Source: CAD feature listing. Evaluate the final solid. Frame: model axes, mm. A direction names the side the tool comes from. Round coordinates to 2 decimals unless told otherwise and drop trailing zeros. Loops run counter-clockwise (first coordinate to the right, second up) from the corner with the lowest first, then second, coordinate; pieces in that order, holes last. Notation, with made-up numbers: (70.5, 82) -> (127.5, 82) arc R20 cw to (127.5, 99) -> close; hole circle Ø1 at (48, 49.25). An arc over 180 degrees is marked (long way). Write item = value, one per line.
from build123d import *

# Parameters (mm, degrees)
F0_W     = 100
F0_H     = 300
F1_DEPTH = 6.35
F2_W     = 2
F2_H     = 40
F3_DEPTH = 25.4


# Not quite as in the source:
# - a length typed as a fraction of an inch, garbled in the dataset ("3 / 203.2 mm" for 3/8 in), is restored


with BuildPart() as f1:
    # F0 (on Top) → F1 (new body)
    with BuildSketch(Plane.XY):
        Rectangle(F0_W, F0_H)
    extrude(amount=F1_DEPTH)

    # F2 (on face) → F3 (cut)
    with BuildSketch(Plane.XY.offset(6.35)):
        Polygon((22.5, 22.48), (22.5, 110.5), (-22.5, 110.5), (-22.5, 22.48), (-22.5, -17.52), (-22.5, -110.5), (22.5, -110.5), (22.5, -17.52), align=None)
        with Locations((23.5, 2.48)):
            Rectangle(F2_W, F2_H)
        with Locations((-23.5, 2.48)):
            Rectangle(F2_W, F2_H)
    extrude(amount=-F3_DEPTH, mode=Mode.SUBTRACT)


solid = f1.part
1. Contact query for a flat-ended pin moving along its axis: pin 1 Ø1.5 at (x, y) = (22.5, 17) entering from -Z. Output: stop coordinate, or through.
Evaluation:
pin_1 = through
2. Section query C-C (z = 4). Return the cut outline in (x, y).
Evaluation:
outline = (-50, -150) -> (50, -150) -> (50, 150) -> (-50, 150) -> close; hole (-24.5, -17.52) -> (-22.5, -17.52) -> (-22.5, -110.5) -> (22.5, -110.5) -> (22.5, -17.52) -> (24.5, -17.52) -> (24.5, 22.48) -> (22.5, 22.48) -> (22.5, 110.5) -> (-22.5, 110.5) -> (-22.5, 22.48) -> (-24.5, 22.48) -> close
3. Section query B-B (y = 37). Return the cut outline in (x, z), then the cut area to 3 significant figures.
Evaluation:
outline = (-50, 0) -> (-22.5, 0) -> (-22.5, 6.35) -> (-50, 6.35) -> close; (22.5, 0) -> (50, 0) -> (50, 6.35) -> (22.5, 6.35) -> close
area = 349 mm²
4. Mould query, pull axis X, two halves, no side actions, for faces 1 (the face through (50, -2, 3)), 2 (the face through (-34, 2, 0)), 3 (the face through (-22.5, 67, 3)). Classes: released by +X, released by -X, zero draft, split by the parting line, or undercut.
Evaluation:
face_1 = released by +X
face_2 = zero draft
face_3 = undercut
5. Line query: probe 1 along X at (y, z) = (-91, 4.75); probe 2 along Y at (x, z) = (20.5, 0.5); probe 3 along X at (y, z) = (16.5, 4.25). Output: solid intervals per line, ascending. Write a range as from..to.
Evaluation:
probe_1 = -50..-22.5, 22.5..50
probe_2 = -150..-110.5, 110.5..150
probe_3 = -50..-24.5, 24.5..50
6. Section query A-A (x = -2). Return the cut outline in (y, z).
Evaluation:
outline = (-150, 0) -> (-110.5, 0) -> (-110.5, 6.35) -> (-150, 6.35) -> close; (110.5, 0) -> (150, 0) -> (150, 6.35) -> (110.5, 6.35) -> close
7. Set-up query: faces 4 (the face through (0, -110.5, 3)), 5 (the face through (-34, 2, 6.35)). Return all of +Z, -Z, +X, -X, +Y, -Y with unobstructed straight access to the full face (end or side cutting, diameter ignored); none if empty.
Evaluation:
face_4 = +Z, -Z
face_5 = +Z, +X, -X, +Y, -Y
